Check sheet for the modelled part. Datum: model origin and axes. Units: mm. Face numbers are marked on the shaded views. Round coordinates to 2 decimals unless told otherwise and drop trailing zeros. Write each loop counter-clockwise with the first axis right and the second up, starting at its lowest first coordinate (ties: lowest second). Pieces come first, ordered by that corner, then holes.
Item 1: Cross-section at A-A on y = -3.5. Enter the section's corners in (x, z) (3 decimals), plus the area to 3 significant figures.
Item 2: Material ranges on line 1 (Z direction, x = 0, y = 0) (3 decimals); line 2 (Z direction, x = 2, y = 2.25) (3 decimals); line 3 (X direction, y = -5.5, z = 2.5), recorded low to high.
Item 3: Go/stop test with flat-tipped pins: pin 1 Ø1 at (y, z) = (6, 7) entering from +X; pin 2 Ø12 at (x, z) = (0, 0) entering from +Y; pin 3 Ø2 at (y, z) = (7, 11.5) entering from -X. Record where each tip stops, or that it passes through.
Item 4: Release check for a two-part mould opening along X. For the marked faces 1, 2, 3 and 4 record: +X half, -X half, draft (parallel to the pull), parting line (faces both ways), or undercut.
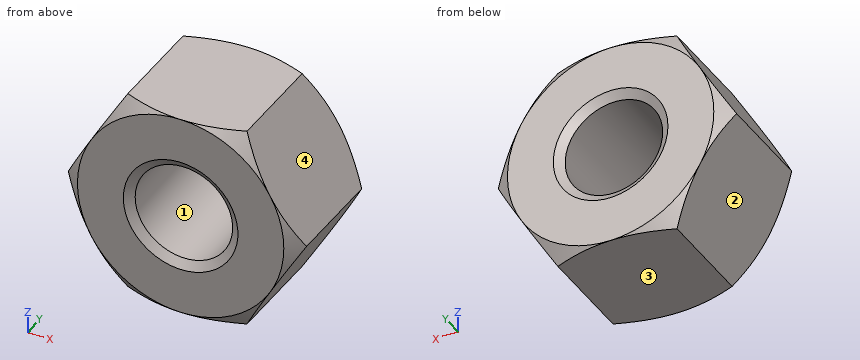
Autodesk Inventor part; units mm, degrees
ref_plane "YZ Plane" through (0, 0, 0) normal (1, 0, 0) x (0, 1, 0)
ref_plane "XZ Plane" through (0, 0, 0) normal (0, 1, 0) x (-1, 0, 0)
ref_plane "XY Plane" through (0, 0, 0) normal (0, 0, 1) x (1, 0, 0)
sketch "Sketch1" plane through (0, 0, 0) normal (0, 1, 0) x (-1, 0, 0)
  line L0 (9.1654, 15.875) -> (18.3309, 0)
  line L1 (18.3309, 0) -> (9.1654, -15.875)
  line L2 (9.1654, -15.875) -> (-9.1654, -15.875)
  line L3 (-9.1654, -15.875) -> (-18.3309, 0)
  line L4 (-18.3309, 0) -> (-9.1654, 15.875)
  line L5 (-9.1654, 15.875) -> (9.1654, 15.875)
  circle A0 centre (0, 0) radius 7.5
  dimension "HEX_FLATS" = 31.75
  dimension "NUT_SIZE" = 15
extrude "Extrusion1" add sketch "Sketch1" along normal mid plane 19.2532
sketch "Sketch2" plane through (0, 0, 0) normal (0, 0, 1) x (1, 0, 0)
  line L0 (18.3309, -9.6266) -> (9.1654, -9.6266)
  line L1 (15.875, -9.6266) -> (18.3309, -7.7216)
  line L2 (28.575, -7.7216) -> (28.575, -20.4216)
  line L3 (28.575, -20.4216) -> (15.875, -20.4216)
  line L4 (15.875, -20.4216) -> (15.875, -9.6266)
  line L5 (0, 0) -> (0, -1.2828)
  line L6 (18.3309, 9.6266) -> (18.3309, -9.6266)
  line L7 (18.3309, -7.7216) -> (28.575, -7.7216)
  line L8 (18.3309, 0) -> (27.089, 0) construction
  dimension "OUTSIDE_CHAMFER_LONG" = 15.875
  dimension "OUTSIDE_CHAMFER_SHORT" = 1.905
  dimension "d12" = 12.7
  dimension "d13" = 12.7
revolve "Revolution1" cut sketch "Sketch2" angle 360 about axis through (0, 0, 0) along (0, -1, 0)
mirror "Mirror1" about plane through (0, 0, 0) normal (0, 1, 0) of "Revolution1"
chamfer "Chamfer1" distance 1.3208 angle 35 1 edges at (7.5, 9.6266, 0) measured on face at (8.9141, 9.6266, 9.4797)
chamfer "Chamfer2" distance 1.3208 angle 35 1 edges at (7.5, -9.6266, 0) measured on face at (8.9141, -9.6266, 9.4797)
properties material "Stainless Steel"
Response values:
1. outline: (-18.331, 0) - (-9.165, -15.875) - (9.165, -15.875) - (18.331, 0) - (9.165, 15.875) - (-9.165, 15.875) - close; hole circle Ø15 at (0, 0)
1. area: 696 mm2
2. line 1: z = -15.875 to -7.5, 7.5 to 15.875
2. line 2: z = -15.875 to -7.228, 7.228 to 15.875
2. line 3: x = -16.89 to -7.07, 7.07 to 16.89
3. pin 1: stops at x = 14.58
3. pin 2: passes through
3. pin 3: stops at x = -12.27
4. face 1: undercut
4. face 2: -X half
4. face 3: draft
4. face 4: +X half
